Verification items for the finished model (mm, model axes). A direction names the side the tool comes from. Coordinates: 2 decimals unless noted, no trailing zeros. Loops run counter-clockwise (first coordinate to the right, second up) from the corner with the lowest first, then second, coordinate; pieces in that order, holes last. Notation, with made-up numbers: (18, 25) - (50, 25) arc R21 ccw to (50, 49) - close; hole circle Ø10 at (-15, -22). An arc over 180 degrees is marked (long way). Answer as CSV lines item,"result". Start each with the question number.
1. Cross-section at B-B (x = 159). Enter the section's corners in (y, z), plus the area to 3 significant figures.
2. Release check for a two-part mould opening along Z. For faces 1 (the flat face through (7, -1, 63)), 2 (the flat face through (157, -1, 128.3)), 3 (the flat face through (158.7, -10, 121.5)) record: pulls with the +Z half, pulls with the -Z half, needs draft (parallel to the pull), parting line crosses it, or undercut.
3. Cross-section at A-A (z = 112). Enter the section's corners in (x, y), plus the area to 3 significant figures.
4. Cross-section at C-C (x = 41.5). Enter the section's corners in (y, z).
5. Cross-section at D-D (z = 39). Enter the section's corners in (x, y), plus the area to 3 significant figures.
6. Gauge pin test, flat end, axial feed: P1, Ø8, axis at y = 6, z = 15.5, coming from the -X side. Record the tip position at first contact, or that the pin passes through.
7. Material ranges on line 1 (X direction, y = 6.75, z = 111); line 2 (Z direction, x = 230, y = -2), recorded low to high. Write a range as [from, to].
8. Set-up check for faces 4 (the flat face through (160, -2.4, 3)), 5 (the flat face through (157, -1, 121.3)), 6 (the flat face through (158.7, 8, 6.8)): record each of +Z, -Z, +X, -X, +Y, -Y from which the full face is reachable in a straight line by a thin tool's end or side.
```python
from build123d import *

# Parameters (mm, degrees)
SKETCH1_W           = 318.8
SKETCH1_H           = 128.3
SKETCH1_W_2         = 304.8
SKETCH1_H_2         = 114.3
BOSS_EXTRUDE1_DEPTH = 8
SKETCH2_W           = 110
SKETCH2_H           = 3
SKETCH2_W_2         = 3
SKETCH2_H_2         = 88.3
CUT_EXTRUDE1_DEPTH  = 3
CHAMFER1_SIZE       = 3
SKETCH3_W           = 318.8
SKETCH3_H           = 128.3
SKETCH3_W_2         = 304.8
SKETCH3_H_2         = 114.3
BOSS_EXTRUDE3_DEPTH = 10
SKETCH4_W           = 15
SKETCH4_H           = 2
CUT_EXTRUDE3_DEPTH  = 7


with BuildPart() as part:
    # Sketch1 → Boss-Extrude1 (new body)
    with BuildSketch(Plane(origin=(0, 0, 0), x_dir=(1, 0, 0), z_dir=(0, 1, 0))):
        with Locations((159.4, -64.15)):
            Rectangle(SKETCH1_W, SKETCH1_H)
        with Locations((159.4, -64.15)):
            Rectangle(SKETCH1_W_2, SKETCH1_H_2, mode=Mode.SUBTRACT)
    extrude(amount=BOSS_EXTRUDE1_DEPTH)

    # Sketch2 → Cut-Extrude1 (cut)
    with BuildSketch(Plane.XZ):
        with Locations((75, 122.8)):
            Rectangle(SKETCH2_W, SKETCH2_H)
        with Locations((5.5, 64.15)):
            Rectangle(SKETCH2_W_2, SKETCH2_H_2)
        with Locations((313.3, 64.15)):
            Rectangle(SKETCH2_W_2, SKETCH2_H_2)
        with Locations((75, 5.5)):
            Rectangle(SKETCH2_W, SKETCH2_H)
        with Locations((243.8, 5.5)):
            Rectangle(SKETCH2_W, SKETCH2_H)
        with Locations((243.8, 122.8)):
            Rectangle(SKETCH2_W, SKETCH2_H)
    extrude(amount=-CUT_EXTRUDE1_DEPTH, mode=Mode.SUBTRACT)

    # Chamfer1
    chamfer1_edges = [part.edges().sort_by_distance(p)[0] for p in [
        (298.8, 1.5, 4),
        (314.8, 1.5, 20),
        (130, 1.5, 4),
        (188.8, 1.5, 4),
        (20, 1.5, 4),
        (4, 1.5, 20),
        (4, 1.5, 108.3),
        (314.8, 1.5, 108.3),
        (298.8, 1.5, 124.3),
        (188.8, 1.5, 124.3),
        (130, 1.5, 124.3),
        (20, 1.5, 124.3),
    ]]
    chamfer(chamfer1_edges, length=CHAMFER1_SIZE - 0.0001)  # a hair under: the kernel refuses the full size

    # Sketch3 → Boss-Extrude3 (add)
    with BuildSketch(Plane.XZ):
        with Locations((159.4, 64.15)):
            Rectangle(SKETCH3_W, SKETCH3_H)
        with Locations((159.4, 64.15)):
            Rectangle(SKETCH3_W_2, SKETCH3_H_2, mode=Mode.SUBTRACT)
    extrude(amount=BOSS_EXTRUDE3_DEPTH)

    # Sketch4 → Cut-Extrude3 (cut)
    with BuildSketch(Plane(origin=(0, 0, 0), x_dir=(-1, 0, 0), z_dir=(0, 0, -1))):
        with Locations((-159.4, -1.4)):
            Rectangle(SKETCH4_W, SKETCH4_H)
    extrude(amount=-CUT_EXTRUDE3_DEPTH, mode=Mode.SUBTRACT)


solid = part.part
```
Values follow:
1,outline,"(-10, 0) - (-2.4, 0) - (-2.4, 7) - (-10, 7) - close; (-10, 121.3) - (8, 121.3) - (8, 128.3) - (-10, 128.3) - close; (-0.4, 0) - (8, 0) - (8, 7) - (-0.4, 7) - close"
1,area,"238 mm²"
2,face 1,"undercut"
2,face 2,"pulls with the +Z half"
2,face 3,"needs draft"
3,outline,"(0, -10) - (7, -10) - (7, 8) - (0, 8) - close; (311.8, -10) - (318.8, -10) - (318.8, 8) - (311.8, 8) - close"
3,area,"252 mm²"
4,outline,"(-10, 0) - (8, 0) - (8, 7) - (3, 7) - (3, 4) - (0, 4) - (0, 7) - (-10, 7) - close; (-10, 121.3) - (0, 121.3) - (0, 124.3) - (3, 124.3) - (3, 121.3) - (8, 121.3) - (8, 128.3) - (-10, 128.3) - close"
5,outline,"(0, -10) - (7, -10) - (7, 0) - (4, 0) - (4, 3) - (7, 3) - (7, 8) - (0, 8) - close; (311.8, -10) - (318.8, -10) - (318.8, 8) - (311.8, 8) - (311.8, 3) - (314.8, 3) - (314.8, 0) - (311.8, 0) - close"
5,area,"234 mm²"
6,P1,"stops at x = 0"
7,line 1,"x = [0, 7], [311.8, 318.8]"
7,line 2,"z = [0, 7], [121.3, 128.3]"
8,face 4,"-Z"
8,face 5,"+Y, -Y"
8,face 6,"+Z, -Z, +X, -X, +Y"
